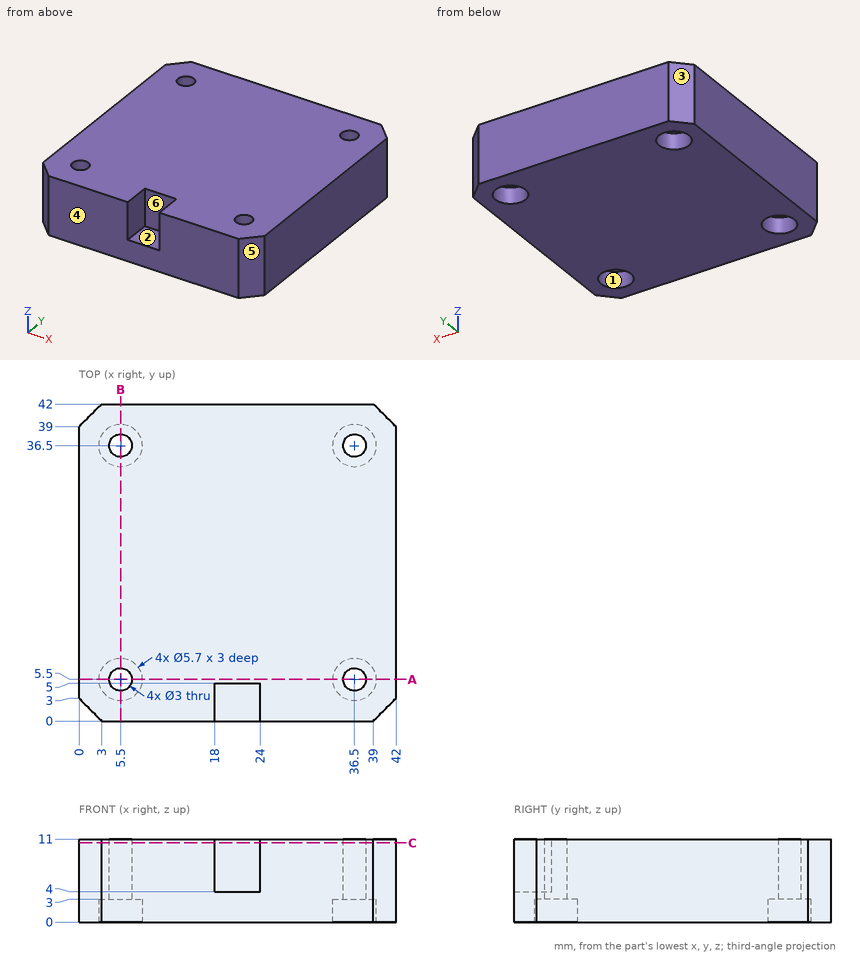
For this review, use the dimensioned drawing (mm, ordinates from the lowest corner) and the shaded views. A direction names the side the tool comes from. Round coordinates to 2 decimals unless told otherwise and drop trailing zeros. Write each loop counter-clockwise with the first axis right and the second up, starting at its lowest first coordinate (ties: lowest second). Pieces come first, ordered by that corner, then holes. Notation, with made-up numbers: M 70.5,-27.75 L 79.5,-27.75 A15 cw 79.5,-23.75 Z; hole C 20.5,28.5 d7. An arc over 180 degrees is marked long. Write item = value, one per line. Start each with the question number.
(1) We need section C-C (z = 10.5). Give the boundary of the cut face in (x, y).
(2) We need section A-A (y = 5.5). Give the boundary of the cut face in (x, z), then the cut area to 3 significant figures.
(3) For line 1 along Y through (x, z) = (36.5, 2); line 2 along X through (y, z) = (3.5, 10); line 3 along X through (y, z) = (37, 7), list the stretches that pass through material, from the lowest coordinate up.
(4) For the marked faces 1, 2 and 3, list the 3-axis set-ups (+Z, -Z, +X, -X, +Y, -Y) from which the entire face can be reached by the end or side of a thin tool; tool diameter is ignored.
(5) Clearance check with flat-ended pins moving along their axes: pin 1 Ø2.5 at (x, y) = (20.5, 3) entering from +Z; pin 2 Ø1.7 at (x, y) = (36.5, 4.5) entering from -Z. State where each tip first meets the part, or that it passes through.
(6) The part is to be moulded in two halves that separate along X. For the marked faces 4, 5 and 6, say which applies: +X half, -X half, draft (parallel to the pull), parting line (faces both ways), or undercut.
Results found:
q1.outline = M 0,3 L 3,0 L 18,0 L 18,5 L 24,5 L 24,0 L 39,0 L 42,3 L 42,39 L 39,42 L 3,42 L 0,39 Z; hole C 5.5,5.5 d3; hole C 5.5,36.5 d3; hole C 36.5,5.5 d3; hole C 36.5,36.5 d3
q2.outline = M 0,0 L 2.65,0 L 2.65,3 L 4,3 L 4,11 L 0,11 Z; M 7,3 L 8.35,3 L 8.35,0 L 33.65,0 L 33.65,3 L 35,3 L 35,11 L 7,11 Z; M 38,3 L 39.35,3 L 39.35,0 L 42,0 L 42,11 L 38,11 Z
q2.area = 380 mm²
q3.line_1 = 0 to 2.65, 8.35 to 33.65, 39.35 to 42
q3.line_2 = 0 to 18, 24 to 42
q3.line_3 = 0 to 4.09, 6.91 to 35.09, 37.91 to 42
q4.face_1 = -Z
q4.face_2 = +Z, -Y
q4.face_3 = +Z, -Z, -X, +Y
q5.pin_1 = 4
q5.pin_2 = 3
q6.face_4 = draft
q6.face_5 = +X half
q6.face_6 = undercut
